Geometry check sheet. Reference: the model listing, model coordinates, mm. A direction names the side the tool comes from. Coordinates: 2 decimals unless noted, no trailing zeros. Write each loop counter-clockwise with the first axis right and the second up, starting at its lowest first coordinate (ties: lowest second). Pieces come first, ordered by that corner, then holes. Notation, with made-up numbers: (49.25, -20) -> (96.25, -20) arc R25 cw to (96.25, 5) -> close; hole circle Ø5 at (24, 42.25). An arc over 180 degrees is marked (long way). Answer in a Markdown table with one row per item. Add a question column.
Q1. Thickness scan on line 1 (X direction, y = -7, z = 0) (1 decimal); line 2 (Y direction, x = 35.5, z = -18); line 3 (Y direction, x = 24, z = -9). Record the ranges inside material, lowest first.
Q2. Gauge pin test, flat ends, axial feed: P1, Ø8, axis at y = -3.5, z = -9, coming from the +X side; P2, Ø4, axis at x = 34, y = 1.5, coming from the -Z side; P3, Ø3, axis at y = -13.5, z = 0.5, coming from the -X side (3 decimals). Record the tip position at first contact, or that the pin passes through.
Q3. Release check for a two-part mould opening along Z. For faces 3 (the face through (4.8, -23.47, 26.77)), 4 (the face through (4.658, -23.467, -26.797)), 5 (the face through (16, -5, 4.457)) record: pulls with the +Z half, pulls with the -Z half, needs draft (parallel to the pull), parting line crosses it, or undercut.
Q4. Tool access check on faces 1 (the face through (18.529, -5, 0)), 2 (the face through (11, -24.46, -11)). Record the directions out of +Z, -Z, +X, -X, +Y, -Y that give a thin tool (end or side, any length) a straight path to the whole face; none if there is none.
Q5. Section check B-B, the plane z = -2.5. Count the separate pieces of the cut face and the enclosed holes in it, and give its area (3 significant figures).
Q6. Section check C-C, the plane x = 32.5. Record the boundary of the cut face in (y, z).
```python
from build123d import *

# Parameters (mm, degrees)
F1_DEPTH    = 15.7734
F3_DEPTH    = 24.4602
F4_T1_DEPTH = 37.9988318329
F4_T3_DEPTH = 37.9988318329
F4_T6_ANGLE = 213.1574660215
F4_T8_ANGLE = 173.1044855741
F6_DEPTH    = 40.2346
F7_R        = 10.16
F8_DEPTH    = 15.7744


# Not quite as in the source:
# - a fillet or chamfer that OpenCascade refuses, or shapes differently, is made with other operations: its cross-section is extruded or revolved along the edge and cut away or added


with BuildPart() as f1:
    # F0 (on Front) → F1 (new body)
    with BuildSketch(Plane.XZ):
        with BuildLine():
            Line((53.975, 19.05), (9.780704698, 26.8489932886))
            Line((9.780704698, 26.8489932886), (0, 28.575))
            ThreePointArc((0, 28.575), (-28.575, 0), (0, -28.575))
            Line((0, -28.575), (9.780704698, -26.8489932886))
            Line((9.780704698, -26.8489932886), (53.975, -19.05))
            ThreePointArc((53.975, -19.05), (73.025, 0), (53.975, 19.05))
        make_face()
    extrude(amount=-F1_DEPTH)

    # F2 (on face) → F3 (join)
    with BuildSketch(Plane.XZ):
        with BuildLine():
            Line((9.780704698, 26.8489932886), (0, 28.575))
            ThreePointArc((0, 28.575), (-28.575, 0), (0, -28.575))
            Line((0, -28.575), (9.780704698, -26.8489932886))
            ThreePointArc((9.780704698, -26.8489932886), (23.4095521288, -16.3866864902), (28.575, 0))
            ThreePointArc((28.575, 0), (23.4095521288, 16.3866864902), (9.780704698, 26.8489932886))
        make_face()
    extrude(amount=F3_DEPTH)

    # F4: fillet of radius 3.302 on 4 edges, made by hand

    # F4_s2 → F4_t1 (cut)
    with BuildSketch(Plane(origin=(-18.7103124217, 0, -3.3018198391), x_dir=(0, 1, 0), z_dir=(0.9847835588, 0, 0.1737853339))):
        with BuildLine():
            ThreePointArc((-21.1582, -28.1401901932), (-23.4930665915, -27.1730567847), (-24.4602, -24.8381901932))
            Line((-24.4602, -24.8381901932), (-24.4602, -28.1401901932))
            Line((-24.4602, -28.1401901932), (-21.1582, -28.1401901932))
        make_face()
    extrude(amount=F4_T1_DEPTH, mode=Mode.SUBTRACT)

    # F4_s4 → F4_t3 (cut)
    with BuildSketch(Plane(origin=(18.7103124217, 0, -3.3018198391), x_dir=(0, 1, 0), z_dir=(-0.9847835588, 0, 0.1737853339))):
        with BuildLine():
            ThreePointArc((-21.1582, -28.1401901932), (-23.4930665915, -27.1730567847), (-24.4602, -24.8381901932))
            Line((-24.4602, -24.8381901932), (-24.4602, -28.1401901932))
            Line((-24.4602, -28.1401901932), (-21.1582, -28.1401901932))
        make_face()
    extrude(amount=F4_T3_DEPTH, mode=Mode.SUBTRACT)

    # F4_s5 → F4_t6 (revolve, cut)
    with BuildSketch(Plane(origin=(0, 0, 0), x_dir=(0, 1, 0), z_dir=(0.95842855, 0, -0.2853326385))):
        with BuildLine():
            ThreePointArc((-24.4602, 25.273), (-23.4930665915, 27.6078665915), (-21.1582, 28.575))
            Line((-21.1582, 28.575), (-24.4602, 28.575))
            Line((-24.4602, 28.575), (-24.4602, 25.273))
        make_face()
    revolve(axis=Axis((0, -24.4602, 0), (0, -1, 0)), revolution_arc=F4_T6_ANGLE, mode=Mode.SUBTRACT)

    # F4_s7 → F4_t8 (revolve, cut)
    with BuildSketch(Plane(origin=(0, 0, 0), x_dir=(0, 1, 0), z_dir=(-0.9981900481, 0, 0.0601384063))):
        with BuildLine():
            ThreePointArc((-21.1582, -28.575), (-23.4930665915, -27.6078665915), (-24.4602, -25.273))
            Line((-24.4602, -25.273), (-24.4602, -28.575))
            Line((-24.4602, -28.575), (-21.1582, -28.575))
        make_face()
    revolve(axis=Axis((0, -24.4602, 0), (0, 1, 0)), revolution_arc=F4_T8_ANGLE, mode=Mode.SUBTRACT)

    # F5 (on face) → F6 (cut, through all)
    with BuildSketch(Plane.XZ.offset(24.4602)):
        with BuildLine():
            Line((18.5293, 4.4565453057), (13.574677167, 4.4565453057))
            ThreePointArc((13.574677167, 4.4565453057), (-14.2821064756, 0.3925440984), (13.3093916754, -5.1954546943))
            Line((13.3093916754, -5.1954546943), (18.5293, -5.1954546943))
            Line((18.5293, -5.1954546943), (18.5293, 4.4565453057))
        make_face()
    extrude(amount=-F6_DEPTH, mode=Mode.SUBTRACT)

    # F7 (on face) → F8 (cut, through all)
    with BuildSketch(Plane.XZ):
        with Locations((56.261, 0)):
            Circle(F7_R)
    extrude(amount=-F8_DEPTH, mode=Mode.SUBTRACT)


solid = f1.part
```
Calculated:
| question | item | result |
|---|---|---|
| 1 | line 1 | x = -28.6 to -14.3, 18.5 to 28.6 |
| 1 | line 2 | y = 0 to 15.77 |
| 1 | line 3 | y = -24.44 to 15.77 |
| 2 | P1 | stops at x = 71.67 |
| 2 | P2 | stops at z = -22.93 |
| 2 | P3 | stops at x = -28.575 |
| 3 | face 3 | pulls with the +Z half |
| 3 | face 4 | pulls with the -Z half |
| 3 | face 5 | undercut |
| 4 | face 1 | +Y, -Y |
| 4 | face 2 | +Z, -Z, +X, -X, -Y |
| 5 | separate pieces | 3 |
| 5 | enclosed holes | 0 |
| 5 | area | 1,360 mm² |
| 6 | outline | (0, -22.84) -> (15.77, -22.84) -> (15.77, 22.84) -> (0, 22.84) -> close |
